```python
from build123d import *

# Parameters (mm, degrees)
SKETCH1_W           = 79.2
SKETCH1_H           = 79.2
BOSS_EXTRUDE1_DEPTH = 3
SKETCH2_W           = 79.2
SKETCH2_H           = 79.2
SKETCH2_W_2         = 77.5
SKETCH2_H_2         = 77.5
BOSS_EXTRUDE2_DEPTH = 25.4
SKETCH3_R           = 3.25
CUT_EXTRUDE2_DEPTH  = 0.85
SKETCH5_W           = 9.525
SKETCH5_H           = 12.7
CUT_EXTRUDE3_DEPTH  = 19.05
SKETCH6_R           = 3.175
SKETCH6_W           = 1
SKETCH6_H           = 65
BOSS_EXTRUDE3_DEPTH = 11.4
SKETCH7_W           = 12.7
SKETCH7_H           = 12.7
CUT_EXTRUDE5_DEPTH  = 26


with BuildPart() as part:
    # Sketch1 → Boss-Extrude1 (new body)
    with BuildSketch(Plane(origin=(0, 0, 0), x_dir=(1, 0, 0), z_dir=(0, 1, 0))):
        Rectangle(SKETCH1_W, SKETCH1_H)
    extrude(amount=BOSS_EXTRUDE1_DEPTH)

    # Sketch2 → Boss-Extrude2 (add)
    with BuildSketch(Plane(origin=(0, 3, 0), x_dir=(1, 0, 0), z_dir=(0, 1, 0))):
        Rectangle(SKETCH2_W, SKETCH2_H)
        Rectangle(SKETCH2_W_2, SKETCH2_H_2, mode=Mode.SUBTRACT)
    extrude(amount=BOSS_EXTRUDE2_DEPTH)

    # Sketch3 → Cut-Extrude2 (cut)
    with BuildSketch(Plane(origin=(39.6, 0, 0), x_dir=(0, 0, -1), z_dir=(1, 0, 0))):
        with Locations((-15.1, 6.35)):
            Circle(SKETCH3_R)
        with BuildLine():
            ThreePointArc((-18.35, 6.35), (-15.1, 9.6), (-11.85, 6.35))
            Line((-11.85, 6.35), (-11.85, 28.4))
            Line((-11.85, 28.4), (-18.35, 28.4))
            Line((-18.35, 28.4), (-18.35, 6.35))
        make_face()
    extrude(amount=-CUT_EXTRUDE2_DEPTH, mode=Mode.SUBTRACT)

    # Sketch5 → Cut-Extrude3 (cut)
    with BuildSketch(Plane.XY.offset(39.6)):
        with Locations((31.8375, 9.35)):
            Rectangle(SKETCH5_W, SKETCH5_H)
        with Locations((-31.8375, 9.35)):
            Rectangle(SKETCH5_W, SKETCH5_H)
    extrude(amount=-CUT_EXTRUDE3_DEPTH, mode=Mode.SUBTRACT)

    # Sketch6 → Boss-Extrude3 (add)
    with BuildSketch(Plane(origin=(0, 3, 0), x_dir=(1, 0, 0), z_dir=(0, 1, 0))):
        with Locations(Location((10.175, 19.7, 0), (0, 0, 90))):
            Circle(SKETCH6_R)
        with Locations((-38.25, 6.25)):
            Rectangle(SKETCH6_W, SKETCH6_H)
    extrude(amount=BOSS_EXTRUDE3_DEPTH)

    # Sketch7 → Cut-Extrude5 (cut)
    with BuildSketch(Plane(origin=(0, 3, 0), x_dir=(1, 0, 0), z_dir=(0, 1, 0))):
        with Locations((8.5875, -11.7625)):
            Rectangle(SKETCH7_W, SKETCH7_H)
    extrude(amount=-CUT_EXTRUDE5_DEPTH, mode=Mode.SUBTRACT)


solid = part.part
```
Build history of the part. All positions in model axes, mm. A direction names the side the tool comes from. Round coordinates to 2 decimals unless told otherwise and drop trailing zeros. Loops run counter-clockwise (first coordinate to the right, second up) from the corner with the lowest first, then second, coordinate; pieces in that order, holes last.
Item 1: Drill centre lines: line 1 along Z through (x, y) = (-6.5, 15.5); line 2 along X through (y, z) = (7.75, 23). Where is each one in solid material? Low to high.
Item 2: Saw through at C-C (y = 13.25). List the corners of the cut face in (x, z) (3 decimals), then the cut area to 3 significant figures.
Item 3: Pin check, flat tips, straight feed: P1, Ø1.5, axis at x = -26, z = -27.5, coming from the +Y side; P2, Ø1.9, axis at x = 11, z = -19.5, coming from the +Y side. Stop position of each tip, or through.
Item 4: Saw through at B-B (z = 15.1). List the corners of the cut face in (x, y), then the cut area to 3 significant figures.
Item 5: Saw through at D-D (z = -19.7). List the corners of the cut face in (x, y), then the cut area to 3 significant figures.
Item 6: Two-plate mould, pull along Z, no slides. Class faces 1 (the face through (39.6, 14, 1)), 2 (the face through (-1, 14, -39.6)), 3 (the face through (-1, 16, -38.75)), 4 (the face through (-1, 14, 39.6)): released by +Z, released by -Z, zero draft, split by the parting line, or undercut.
Item 7: Saw through at A-A (x = -31). List the corners of the cut face in (y, z).
Item 8: Which spindle directions (+Z, -Z, +X, -X, +Y, -Y) get a long thin tool onto all of the face, cutting with end or side? Do faces 5 (the face through (38.75, 16, 1)), 6 (the face through (39.2, 3.1, 15.2)), 7 (the face through (14.938, 2, 12)), 8 (the face through (-1, 0, -1)), 9 (the face through (-39.6, 14, 1)). Say none if no direction does.
Worked answers:
1. line 1: z = -39.6 to -38.75, 38.75 to 39.6
1. line 2: x = -39.6 to -37.75, 38.75 to 39.6
2. outline: (-39.6, -39.6) - (39.6, -39.6) - (39.6, 11.85) - (38.75, 11.85) - (38.75, -38.75) - (-37.75, -38.75) - (-37.75, 26.25) - (-38.75, 26.25) - (-38.75, 38.75) - (-36.6, 38.75) - (-36.6, 39.6) - (-39.6, 39.6) - close; (-27.075, 38.75) - (27.075, 38.75) - (27.075, 39.6) - (-27.075, 39.6) - close; circle Ø6.35 at (10.175, -19.7); (36.6, 38.75) - (38.75, 38.75) - (38.75, 18.35) - (39.6, 18.35) - (39.6, 39.6) - (36.6, 39.6) - close
2. area: 341 mm2
3. P1: stops at y = 3
3. P2: stops at y = 14.4
4. outline: (-39.6, 0) - (2.24, 0) - (2.24, 3) - (-37.75, 3) - (-37.75, 14.4) - (-38.75, 14.4) - (-38.75, 28.4) - (-39.6, 28.4) - close; (14.94, 0) - (39.6, 0) - (39.6, 3.1) - (38.75, 3.1) - (38.75, 3) - (14.94, 3) - close
4. area: 233 mm2
5. outline: (-39.6, 0) - (39.6, 0) - (39.6, 28.4) - (38.75, 28.4) - (38.75, 3) - (13.35, 3) - (13.35, 14.4) - (7, 14.4) - (7, 3) - (-37.75, 3) - (-37.75, 14.4) - (-38.75, 14.4) - (-38.75, 28.4) - (-39.6, 28.4) - close
5. area: 365 mm2
6. face 1: zero draft
6. face 2: released by -Z
6. face 3: undercut
6. face 4: released by +Z
7. outline: (0, -39.6) - (28.4, -39.6) - (28.4, -38.75) - (3, -38.75) - (3, 39.6) - (0, 39.6) - close; (15.7, 38.75) - (28.4, 38.75) - (28.4, 39.6) - (15.7, 39.6) - close
8. face 5: +Y
8. face 6: +X, +Y
8. face 7: +Y, -Y
8. face 8: +Z, -Z, +X, -X, -Y
8. face 9: +Z, -Z, -X, +Y, -Y
